Drawing for the job (mm, zero at the part's lowest x, y, z). A direction names the side the tool comes from. Give positions to 0.01 mm unless a question says otherwise; leave off trailing zeros. Write each loop counter-clockwise with the first axis right and the second up, starting at its lowest first coordinate (ties: lowest second). Pieces come first, ordered by that corner, then holes. Notation, with made-up numbers: M 66.25,56.25 L 115.25,56.25 A23 cw 115.25,93.25 Z; hole C 77.5,15.5 d3. An arc over 180 degrees is marked long. Write item = value, one per line. Start each with the question number.
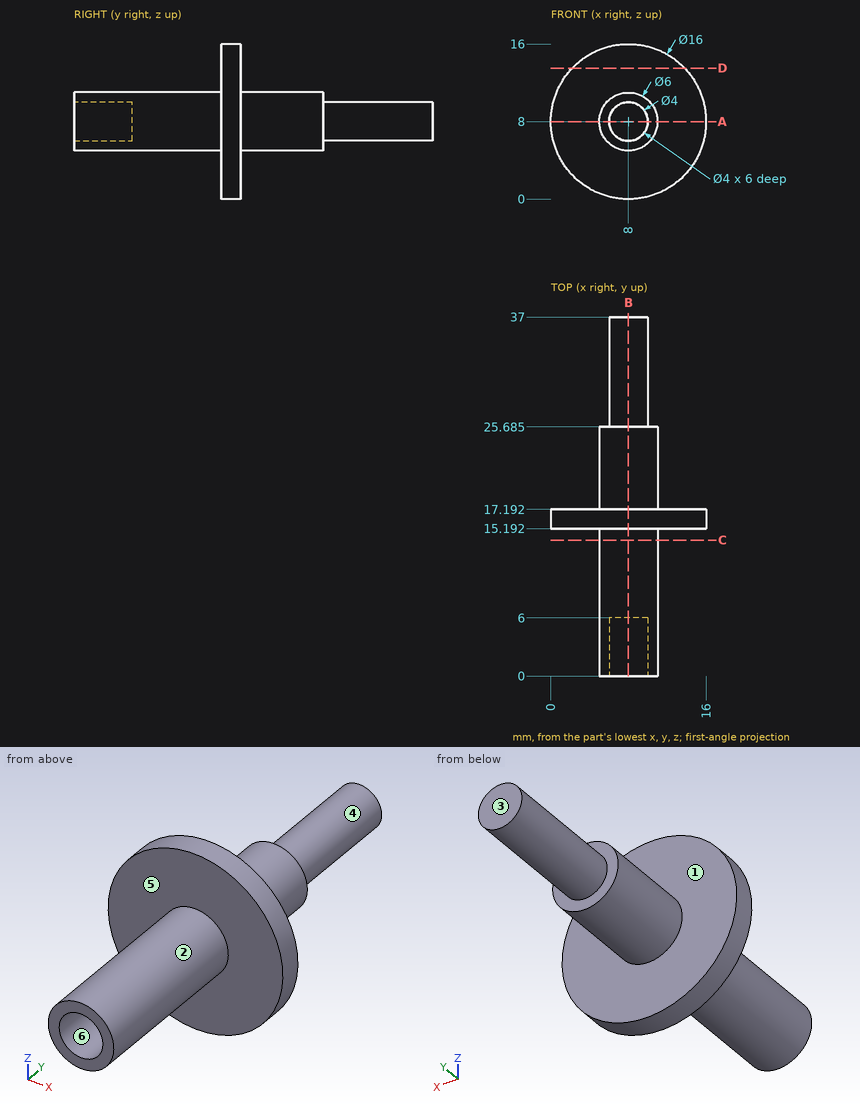
Q1. Two-plate mould, pull along Z, no slides. Class the marked faces 4, 5 and 6: +Z half, -Z half, draft (parallel to the pull), parting line (faces both ways), or undercut.
Q2. Slice it at D-D (z = 13.5). Give the cut face in (x, y).
Q3. Slice it at A-A (z = 8). Give the cut face in (x, y) (1 decimal), and give its area (3 significant figures).
Q4. Slice it at C-C (y = 14). Give the cut face in (x, z).
Q5. Slice it at B-B (x = 8). Give the cut face in (y, z) (1 decimal).
Q6. Probe line 1 along X through (y, z) = (3.4, 8); line 2 along Y through (x, z) = (15.25, 9); line 3 along Z through (x, y) = (13, 17) (1 decimal). List the from-to ranges inside material, lowest first.
Q7. Tool access for the marked faces 1, 2 and 3: list every direction of +Z, -Z, +X, -X, +Y, -Y with a clear straight run to the whole face (end or side of a thin tool).
Q8. Drop flat-ended pins along their axis: P1, Ø5, axis at y = 17, z = 12, coming from the +X side; P2, Ø5, axis at y = 4.5, z = 9, coming from the -X side; P3, Ø3, axis at x = 10, y = 19.5, coming from the -Z side. Give the stop position or say it passes through.
Working result:
q1.face_4 = parting line
q1.face_5 = draft
q1.face_6 = undercut
q2.outline = M 2.19,15.19 L 13.81,15.19 L 13.81,17.19 L 2.19,17.19 Z
q3.outline = M 0,15.2 L 5,15.2 L 5,0 L 6,0 L 6,6 L 10,6 L 10,0 L 11,0 L 11,15.2 L 16,15.2 L 16,17.2 L 11,17.2 L 11,25.7 L 10,25.7 L 10,37 L 6,37 L 6,25.7 L 5,25.7 L 5,17.2 L 0,17.2 Z
q3.area = 195 mm2
q4.outline = C 8,8 d6
q5.outline = M 0,5 L 15.2,5 L 15.2,0 L 17.2,0 L 17.2,5 L 25.7,5 L 25.7,6 L 37,6 L 37,10 L 25.7,10 L 25.7,11 L 17.2,11 L 17.2,16 L 15.2,16 L 15.2,11 L 0,11 L 0,10 L 6,10 L 6,6 L 0,6 Z
q6.line_1 = 5 to 6, 10 to 11
q6.line_2 = 15.19 to 17.19
q6.line_3 = 1.8 to 14.2
q7.face_1 = +Y
q7.face_2 = -Y
q7.face_3 = +Z, -Z, +X, -X, +Y
q8.P1 = 15.86
q8.P2 = 5
q8.P3 = 5.04
